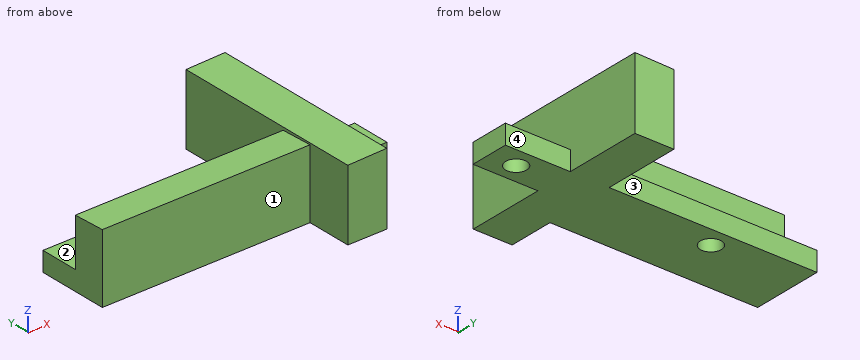
```python
from build123d import *

# Parameters (mm, degrees)
BOSS_EXTRU_1_DEPTH      = 3
ESQUISSE2_R             = 1.625
ENL_V_MAT_EXTRU_1_DEPTH = 4
BOSS_EXTRU_2_DEPTH      = 10
BOSS_EXTRU_2_DEPTH_BACK = 3
ENL_V_MAT_EXTRU_2_DEPTH = 32
ESQUISSE7_W             = 6
ESQUISSE7_H             = 30
ENL_V_MAT_EXTRU_4_DEPTH = 2
ENL_V_MAT_EXTRU_5_DEPTH = 30


with BuildPart() as part:
    # Esquisse1 → Boss.-Extru.1 (new body)
    with BuildSketch(Plane.XY):
        Polygon((32, -6), (32, -18), (38, -18), (38, -6), (48, -6), (48, 0), (38, 0), (38, 12), (32, 12), (32, 0), (0, 0), (0, -6), align=None)
    extrude(amount=BOSS_EXTRU_1_DEPTH)

    # Esquisse2 → Enlèv. mat.-Extru.1 (cut, through all)
    with BuildSketch(Plane.XY.offset(3)):
        with Locations((13.85, -3)):
            Circle(ESQUISSE2_R)
        with Locations((43.85, -3)):
            Circle(ESQUISSE2_R)
    extrude(amount=-ENL_V_MAT_EXTRU_1_DEPTH, mode=Mode.SUBTRACT)

    # Esquisse3 → Boss.-Extru.2 (add, two sides)
    with BuildSketch(Plane.XY.offset(3)) as boss_extru_2_sk:
        Polygon((38, 12), (32, 12), (32, -6), (0, -6), (0, -11), (32, -11), (32, -18), (38, -18), align=None)
    extrude(amount=BOSS_EXTRU_2_DEPTH)
    extrude(boss_extru_2_sk.sketch, amount=-BOSS_EXTRU_2_DEPTH_BACK)

    # Esquisse4 → Enlèv. mat.-Extru.2 (cut)
    with BuildSketch(Plane.ZY):
        Polygon((13, -6), (13, -11), (10.6, -11), (10.4, -6), align=None)
    extrude(amount=-ENL_V_MAT_EXTRU_2_DEPTH, mode=Mode.SUBTRACT)

    # Esquisse7 → Enlèv. mat.-Extru.4 (cut)
    with BuildSketch(Plane.XY.offset(13)):
        with Locations((35, -3)):
            Rectangle(ESQUISSE7_W, ESQUISSE7_H)
    extrude(amount=-ENL_V_MAT_EXTRU_4_DEPTH, mode=Mode.SUBTRACT)

    # Esquisse8 → Enlèv. mat.-Extru.5 (cut)
    with BuildSketch(Plane.XZ.offset(18)):
        Polygon((32, 11), (32, 10.85), (38, 11), align=None)
    extrude(amount=-ENL_V_MAT_EXTRU_5_DEPTH, mode=Mode.SUBTRACT)


solid = part.part
```
Verification items for the finished model (mm, model axes). Face numbers are marked on the shaded views. A direction names the side the tool comes from. Give positions to 0.01 mm unless a question says otherwise; leave off trailing zeros. Loops run counter-clockwise (first coordinate to the right, second up) from the corner with the lowest first, then second, coordinate; pieces in that order, holes last.
1. Go/stop test with flat-tipped pins: pin 1 Ø4 at (x, y) = (35, 7) entering from +Z (3 decimals); pin 2 Ø1.8 at (x, y) = (21, -3) entering from +Z; pin 3 Ø4 at (y, z) = (-1.5, 9) entering from +X. Record where each tip stops, or that it passes through.
2. Section check C-C, the plane y = -0.5. Enter the section's corners in (x, z).
3. Section check D-D, the plane x = 13.85. Enter the section's corners in (y, z) (3 decimals).
4. Section check A-A, the plane x = 43.85. Enter the section's corners in (y, z) (3 decimals).
5. Section check B-B, the plane z = 1.75. Enter the section's corners in (x, y) (3 decimals), then the cut area to 3 significant figures.
6. Thickness scan on line 1 (Y direction, x = 43.85, z = 2.35) (3 decimals); line 2 (Y direction, x = 13.85, z = 2.3) (3 decimals); line 3 (X direction, y = -2.25, z = 2.5). Record the ranges inside material, lowest first.
7. Set-up check for the marked faces 1, 2, 3 and 4: record each of +Z, -Z, +X, -X, +Y, -Y from which the full face is reachable in a straight line by a thin tool's end or side.
Geometry says:
1. pin 1: stops at z = 10.975
1. pin 2: stops at z = 3
1. pin 3: stops at x = 38
2. outline: (0, 0) - (48, 0) - (48, 3) - (38, 3) - (38, 11) - (32, 10.85) - (32, 3) - (0, 3) - close
3. outline: (-11, 0) - (-4.625, 0) - (-4.625, 3) - (-6, 3) - (-6, 10.4) - (-11, 10.6) - close; (-1.375, 0) - (0, 0) - (0, 3) - (-1.375, 3) - close
4. outline: (-6, 0) - (-4.625, 0) - (-4.625, 3) - (-6, 3) - close; (-1.375, 0) - (0, 0) - (0, 3) - (-1.375, 3) - close
5. outline: (0, -11) - (32, -11) - (32, -18) - (38, -18) - (38, -6) - (48, -6) - (48, 0) - (38, 0) - (38, 12) - (32, 12) - (32, 0) - (0, 0) - close; hole circle Ø3.25 at (13.85, -3); hole circle Ø3.25 at (43.85, -3)
5. area: 575 mm2
6. line 1: y = -6 to -4.625, -1.375 to 0
6. line 2: y = -11 to -4.625, -1.375 to 0
6. line 3: x = 0 to 12.41, 15.29 to 42.41, 45.29 to 48
7. face 1: +Z, -Z, -X, -Y
7. face 2: +Z, -X, +Y
7. face 3: +Z, -Z, -X, +Y
7. face 4: +Z, -Z, +X, +Y
